Autodesk Inventor part; units mm, degrees
ref_plane "YZ Plane" through (0, 0, 0) normal (1, 0, 0) x (0, 1, 0)
ref_plane "XZ Plane" through (0, 0, 0) normal (0, 1, 0) x (-1, 0, 0)
ref_plane "XY Plane" through (0, 0, 0) normal (0, 0, 1) x (1, 0, 0)
sketch "スケッチ1" plane through (0, 0, 0) normal (0, 1, 0) x (-1, 0, 0)
  line L0 (234, 0) -> (-39, 0)
  line L1 (0, -180) -> (0, 30)
  line L2 (0, 0) -> (195, 0)
  line L3 (195, 0) -> (195, -150)
  line L4 (175, -20) -> (0, -20)
  circle A0 centre (10, -10) radius 5
  circle A1 centre (185, -110) radius 5
  line L5 (195, -150) -> (175, -150)
  circle A2 centre (185, -140) radius 5
  line L6 (175, -20) -> (175, -150)
  dimension "d0" = 195
  dimension "d2" = 20
  dimension "d3" = 150
  dimension "d5" = 10
  dimension "d6" = 10
  dimension "d7" = 10
  dimension "d8" = 10
  dimension "d9" = 10
  dimension "d23" = 40
  dimension "d24" = 10
  dimension "d30" = 10
  dimension "d31" = 10
  dimension "d34" = 20
extrude "押し出し4" add sketch "スケッチ1" along normal blind 5
properties part number "rocker_alt" material "アルミニウム 6061"
Design review of the part built by this model. Coordinates are the model's own, in mm. A direction names the side the tool comes from. Round coordinates to 2 decimals unless told otherwise and drop trailing zeros. Write each loop counter-clockwise with the first axis right and the second up, starting at its lowest first coordinate (ties: lowest second). Pieces come first, ordered by that corner, then holes. Notation, with made-up numbers: (59, -13) - (77, -13) arc R16 ccw to (77, 5) - close; hole circle Ø8 at (-23, 20). An arc over 180 degrees is marked (long way). Return JSON: item names as keys, results as strings. Group by question number.
Item 1: We need section B-B on z = -110. Write out the cut boundary in (x, y).
Item 2: Insertion check: P1, Ø1, axis at x = -50, y = 1, coming from the +Z side; P2, Ø1.5, axis at x = -104, y = 3.5, coming from the -Z side; P3, Ø6, axis at x = -185, z = -110, coming from the +Y side; P4, Ø1, axis at y = 4, z = -132.5, coming from the +X side. Each pin has a flat end and moves straight along its axis. Give the tip position at first contact, or say it passes through.
Item 3: The part is to be moulded in two halves that separate along X. For faces 1 (the face through (-99, 2, 0)), 2 (the face through (-14.77, 2.46, -11.5)), 3 (the face through (0, 2, -10)), say which applies: pulls with the +X half, pulls with the -X half, needs draft (parallel to the pull), parting line crosses it, or undercut.
Item 4: For probe 1 along Z at (x, y) = (-185, 2.6); probe 2 along Z at (x, y) = (-10, 1.65); probe 3 along X at (y, z) = (1.6, -61.5), list the stretches that pass through material, from the lowest coordinate up. Write a range as [from, to].
Item 5: We need section A-A on x = -185. Write out the cut boundary in (y, z), and give its area (3 significant figures).
Item 6: Machinability: for faces 4 (the face through (-181, 2, -137)), 5 (the face through (-89, 2, -20)), which of the approach directions +Z, -Z, +X, -X, +Y, -Y give a long, thin tool a straight path to every point of the face, cutting with its end or side? Answer none if there is none.
Item 7: We need section D-D on y = 3.45. Write out the cut boundary in (x, z).
Item 8: We need section C-C on x = -10. Write out the cut boundary in (y, z).
Model answer:
{
 "1": {"outline": "(-195, 0) - (-190, 0) - (-190, 5) - (-195, 5) - close; (-180, 0) - (-175, 0) - (-175, 5) - (-180, 5) - close"},
 "2": {"P1": "stops at z = 0", "P2": "stops at z = -20", "P3": "passes through", "P4": "stops at x = -175"},
 "3": {"face 1": "needs draft", "face 2": "undercut", "face 3": "pulls with the +X half"},
 "4": {"probe 1": "z = [-150, -145], [-135, -115], [-105, 0]", "probe 2": "z = [-20, -15], [-5, 0]", "probe 3": "x = [-195, -175]"},
 "5": {"outline": "(0, -150) - (5, -150) - (5, -145) - (0, -145) - close; (0, -135) - (5, -135) - (5, -115) - (0, -115) - close; (0, -105) - (5, -105) - (5, 0) - (0, 0) - close", "area": "650 mm²"},
 "6": {"face 4": "+Y, -Y", "face 5": "-Z, +X, +Y, -Y"},
 "7": {"outline": "(-195, -150) - (-175, -150) - (-175, -20) - (0, -20) - (0, 0) - (-195, 0) - close; hole circle Ø10 at (-185, -140); hole circle Ø10 at (-185, -110); hole circle Ø10 at (-10, -10)"},
 "8": {"outline": "(0, -20) - (5, -20) - (5, -15) - (0, -15) - close; (0, -5) - (5, -5) - (5, 0) - (0, 0) - close"}
}
